For this review, take the finished solid that the model builds, in its own axes (mm). Face numbers are marked on the shaded views. A direction names the side the tool comes from. Round coordinates to 2 decimals unless told otherwise and drop trailing zeros. Order: outer loops, then holes, each group sorted by start corner. A loop starts at its lowest first (then second) coordinate and runs counter-clockwise, first axis right, second up. Notation, with made-up numbers: M -34,82 L -13,82 A31 cw -13,112 Z; hole C 26.5,66.5 d4. An arc over 180 degrees is marked long. Answer as a JSON object with one key per item and string values.
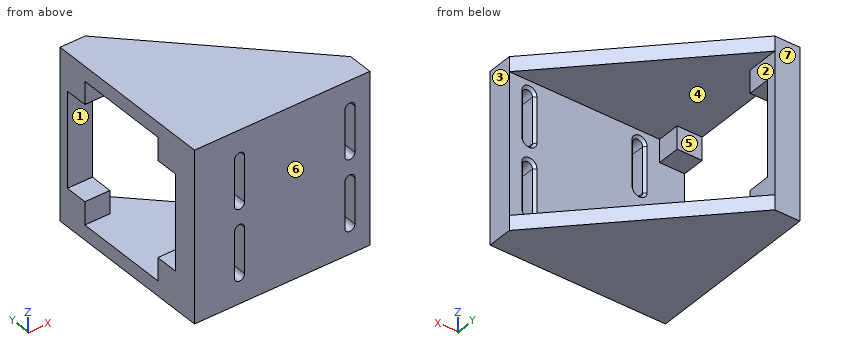
from build123d import *

# Parameters (mm, degrees)
BOSS_EXTRUDE1_DEPTH = 34
CUT_EXTRUDE1_DEPTH  = 28.1
CUT_EXTRUDE2_DEPTH  = 99.264947972
CHAMFER1_SIZE       = 1
CUT_EXTRUDE3_DEPTH  = 79.788387469


with BuildPart() as part:
    # Sketch2 → Boss-Extrude1 (new, symmetric)
    with BuildSketch(Plane.XY):
        Polygon((0, 31.9), (0, -38.1), (70, -38.1), (70, -28.1), (10, 31.9), align=None)
    extrude(amount=BOSS_EXTRUDE1_DEPTH, both=True)

    # Sketch4 → Cut-Extrude1 (cut, symmetric)
    with BuildSketch(Plane.XY):
        Polygon((10, 31.9), (70, -28.1), (10, -28.1), align=None)
    extrude(amount=CUT_EXTRUDE1_DEPTH, both=True, mode=Mode.SUBTRACT)

    # Sketch5 → Cut-Extrude2 (cut, through all)
    with BuildSketch(Plane(origin=(0, -28.1, 0), x_dir=(1, 0, 0), z_dir=(0, 1, 0))):
        with BuildLine():
            Line((20, 23.1), (20, 5))
            ThreePointArc((20, 5), (18, 3), (16, 5))
            Line((16, 5), (16, 23.1))
            ThreePointArc((16, 23.1), (18, 25.1), (20, 23.1))
        make_face()
        with BuildLine():
            Line((64, 23.1), (64, 5))
            ThreePointArc((64, 5), (62, 3), (60, 5))
            Line((60, 5), (60, 23.1))
            ThreePointArc((60, 23.1), (62, 25.1), (64, 23.1))
        make_face()
        with BuildLine():
            Line((64, -23.1), (64, -5))
            ThreePointArc((64, -5), (62, -3), (60, -5))
            Line((60, -5), (60, -23.1))
            ThreePointArc((60, -23.1), (62, -25.1), (64, -23.1))
        make_face()
        with BuildLine():
            Line((20, -23.1), (20, -5))
            ThreePointArc((20, -5), (18, -3), (16, -5))
            Line((16, -5), (16, -23.1))
            ThreePointArc((16, -23.1), (18, -25.1), (20, -23.1))
        make_face()
    extrude(amount=-CUT_EXTRUDE2_DEPTH, mode=Mode.SUBTRACT)

    # Chamfer1
    chamfer1_edges = [part.edges().sort_by_distance(p)[0] for p in [
        (18, -28.1, 25.1),
        (20, -28.1, 14.05),
        (18, -28.1, 3),
        (16, -28.1, 14.05),
        (62, -28.1, 25.1),
        (64, -28.1, 14.05),
        (62, -28.1, 3),
        (60, -28.1, 14.05),
        (62, -28.1, -25.1),
        (60, -28.1, -14.05),
        (62, -28.1, -3),
        (64, -28.1, -14.05),
        (18, -28.1, -25.1),
        (16, -28.1, -14.05),
        (18, -28.1, -3),
        (20, -28.1, -14.05),
    ]]
    chamfer(chamfer1_edges, length=CHAMFER1_SIZE)

    # Sketch6 → Cut-Extrude3 (cut, through all)
    with BuildSketch(Plane(origin=(10, 0, 0), x_dir=(0, 0, -1), z_dir=(1, 0, 0))):
        Polygon((-28.1, 19), (-28.1, -19), (-19, -19), (-19, -28.1), (19, -28.1), (19, -19), (28.1, -19), (28.1, 19), (19, 19), (19, 28.1), (-19, 28.1), (-19, 19), align=None)
    extrude(amount=-CUT_EXTRUDE3_DEPTH, mode=Mode.SUBTRACT)


solid = part.part
1) Insertion check: P1, Ø2, axis at x = 62.5, z = -13, coming from the +Y side; P2, Ø4.5, axis at y = -32, z = 15, coming from the -X side; P3, Ø17, axis at x = 32, z = -7, coming from the +Y side; P4, Ø2.5, axis at y = -24.5, z = 22.5, coming from the +X side. Each pin has a flat end and moves straight along its axis. Give the tip position at first contact, or say it passes through.
Geometry check:
{"P1": "passes through", "P2": "stops at x = 0", "P3": "stops at y = -28.1", "P4": "stops at x = 10"}
2) Add section C-C on z = -12.5. State the section outline as (x, y) points, and give its area (3 significant figures).
Geometry check:
{"outline": "M 0,-38.1 L 16,-38.1 L 16,-29.1 L 15,-28.1 L 0,-28.1 Z; M 0,28.1 L 10,28.1 L 10,31.9 L 0,31.9 Z; M 20,-38.1 L 60,-38.1 L 60,-29.1 L 59,-28.1 L 21,-28.1 L 20,-29.1 Z; M 64,-38.1 L 70,-38.1 L 70,-28.1 L 65,-28.1 L 64,-29.1 Z", "area": "656 mm²"}
3) Add section B-B on x = 62. State the section outline as (y, z) points, and give its area (3 significant figures).
Geometry check:
{"outline": "M -38.1,-34 L -20.1,-34 L -20.1,-28.1 L -28.1,-28.1 L -28.1,-26.1 L -29.1,-25.1 L -38.1,-25.1 Z; M -38.1,-3 L -29.1,-3 L -28.1,-2 L -28.1,2 L -29.1,3 L -38.1,3 Z; M -38.1,25.1 L -29.1,25.1 L -28.1,26.1 L -28.1,28.1 L -20.1,28.1 L -20.1,34 L -38.1,34 Z", "area": "330 mm²"}
4) Add section A-A on y = 25.5. State the section outline as (x, z) points, and give its area (3 significant figures).
Geometry check:
{"outline": "M 0,-34 L 16.4,-34 L 16.4,-28.1 L 10,-28.1 L 10,-19 L 0,-19 Z; M 0,19 L 10,19 L 10,28.1 L 16.4,28.1 L 16.4,34 L 0,34 Z", "area": "376 mm²"}
5) For L1, parallel to X at y = -34, z = -13.5; L2, parallel to Z at x = 18, y = -30; L3, parallel to Z at x = 13, y = 13, list the stretches that pass through material, from the lowest coordinate up.
Geometry check:
{"L1": "x = 0 to 16, 20 to 60, 64 to 70", "L2": "z = -34 to -25.1, -3 to 3, 25.1 to 34", "L3": "z = -34 to -28.1, 28.1 to 34"}
6) Machinability: for the marked faces 1, 2, 3 and 4, which of the approach directions +Z, -Z, +X, -X, +Y, -Y give a long, thin tool a straight path to every point of the face, cutting with its end or side? Answer none if there is none.
Geometry check:
{"face 1": "+X, -X", "face 2": "+X, +Y", "face 3": "+Z, -Z, +X, +Y, -Y", "face 4": "+X"}
7) Add section D-D on x = 24. State the section outline as (y, z) points.
Geometry check:
{"outline": "M -38.1,-34 L 17.9,-34 L 17.9,-28.1 L -28.1,-28.1 L -28.1,28.1 L 17.9,28.1 L 17.9,34 L -38.1,34 Z"}
8) Mouldability with a two-part tool opening along Y and no side actions: class the marked faces 5, 6 and 7 as +Y half, -Y half, draft (parallel to the pull), parting line (faces both ways), or undercut.
Geometry check:
{"face 5": "undercut", "face 6": "-Y half", "face 7": "+Y half"}
